For this review, take the finished solid that the model builds, in its own axes (mm). Face numbers are marked on the shaded views. Coordinates: 2 decimals unless noted, no trailing zeros. Order: outer loops, then holes, each group sorted by start corner. A loop starts at its lowest first (then second) coordinate and runs counter-clockwise, first axis right, second up. Notation, with made-up numbers: M -14.5,-2.75 L 34.5,-2.75 A32 ccw 34.5,29.25 Z; hole C -35.75,58.5 d5. An arc over 180 degrees is marked long. Use CSV: the item, a comma, the result in double quotes.
```python
from build123d import *

# Parameters (mm, degrees)
F1_DEPTH = 8
F3_W     = 8
F3_H     = 8
F3_R     = 2.4
F4_DEPTH = 1.7
F5_R     = 2.4
F6_DEPTH = 1.7


with BuildPart() as f1:
    # F0 (on Front) → F1 (new body)
    with BuildSketch(Plane.XZ):
        Polygon((-2.4, 9.6), (-4, 9.6), (-4, 0), (4, 0), (4, 9.6), (2.4, 9.6), (2.4, 11.3), (-2.4, 11.3), align=None)
    extrude(amount=F1_DEPTH)

    # F3 (on plane+point) → F4 (cut, through all)
    with BuildSketch(Plane.XY.offset(11.3)):
        with Locations((0, -4)):
            Rectangle(F3_W, F3_H)
        with Locations((0, -4)):
            Circle(F3_R, mode=Mode.SUBTRACT)
    extrude(amount=-F4_DEPTH, mode=Mode.SUBTRACT)

    # F5 (on Top) → F6 (cut)
    with BuildSketch(Plane.XY):
        with Locations((0, -4)):
            Circle(F5_R)
    extrude(amount=F6_DEPTH, mode=Mode.SUBTRACT)

    # F8: F1 across plane


with BuildPart() as f1_1:
    add(f1.part)
    add(f1.part.mirror(Plane.YZ.offset(4)))

    # F10: F1 across plane


with BuildPart() as f1_2:
    add(f1_1.part)
    add(f1_1.part.mirror(Plane.YZ.offset(12)))

    # F12: F1 across plane


with BuildPart() as f1_3:
    add(f1_2.part)
    add(f1_2.part.mirror(Plane.YZ.offset(28)))


solid = f1_3.part
```
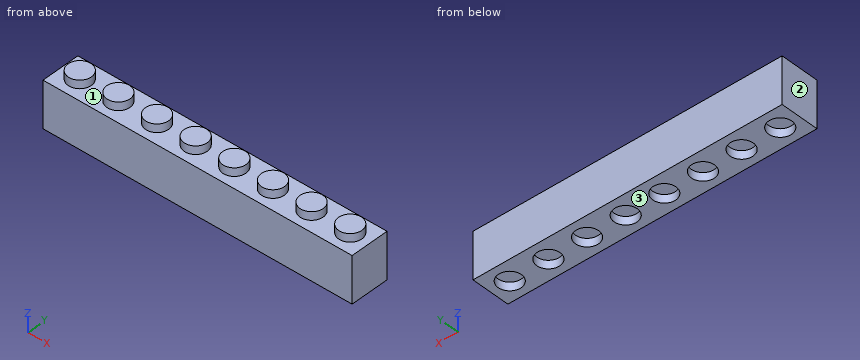
Item 1: Draft analysis for pull direction X (two halves, no side actions). For the marked faces 1, 2 and 3, state which applies: released by +X, released by -X, zero draft, split by the parting line, or undercut.
Solutions:
face 1,"undercut"
face 2,"released by -X"
face 3,"zero draft"
Item 2: To check wall thickness, follow line 1 along Y through (x, z) = (8, 1.2); line 2 along Z through (x, y) = (46, -3.25); line 3 along Z through (x, y) = (34.5, -6.5). State the ranges of each line that lie inside material, in increasing order. Write a range as [from, to].
Solutions:
line 1,"[-8, -6.4], [-1.6, 0]"
line 2,"[1.7, 11.3]"
line 3,"[0, 9.6]"
Item 3: Add section A-A on z = 10.25. State the section outline as (x, y) points.
Solutions:
outline,"C 0,-4 d4.8; C 8,-4 d4.8; C 16,-4 d4.8; C 24,-4 d4.8; C 32,-4 d4.8; C 40,-4 d4.8; C 48,-4 d4.8; C 56,-4 d4.8"
Item 4: Clearance check with a flat-ended pin moving along its axis: pin 1 Ø2 at (x, y) = (40, -4.5) entering from -Z. State where the tip first meets the part, or that it passes through.
Solutions:
pin 1,"z = 1.7"
Item 5: Add section B-B on x = 3.5. State the section outline as (y, z) points.
Solutions:
outline,"M -8,0 L 0,0 L 0,9.6 L -8,9.6 Z"
